Read the model definition and answer for the solid it produces. Units are mm, in the model's axes. A direction names the side the tool comes from. Give positions to 0.01 mm unless a question says otherwise; leave off trailing zeros. Loops run counter-clockwise (first coordinate to the right, second up) from the corner with the lowest first, then second, coordinate; pieces in that order, holes last. Notation, with made-up numbers: (-11.75, 52.5) -> (31.25, 52.5) arc R37 cw to (31.25, 90.5) -> close; hole circle Ø5 at (-34.75, 48). An arc over 180 degrees is marked (long way). Write each question's results on one line, items separated by ' | '. Start each with the question number.
Item 1: Each of these flat-tipped pins is pushed along its axis until it touches: P1, Ø2.5, axis at x = 9.16, y = -37.72, coming from the -Z side; P2, Ø5, axis at x = -6.5, y = -13.5, coming from the -Z side; P3, Ø1.5, axis at y = -6.5, z = 5, coming from the -X side; P4, Ø1.5, axis at y = -25, z = 1.5, coming from the -X side. Where does it stop, or does it pass through?
Item 2: Which of the six approach directions +Z, -Z, +X, -X, +Y, -Y give full straight-line access (tool end or side, diameter ignored) to faces 1 (the flat face through (13.03, 38, 3)), 2 (the cylindrical face through (11.763, -28.375, 2.958))?
Item 3: Section A-A on z = 3.15 is taken. Write down the section's boundary in (x, y), and give its area (3 significant figures).
Item 4: Find the intervals of material crossed by line 1 (Y direction, x = 2.5, z = 3.8); line 2 (Y direction, x = 11, z = 1.1); line 3 (Y direction, x = -7, z = 2.15), in increasing order.
Item 5: Section D-D on x = -4.5 is taken. Write down the section's boundary in (y, z), and give its area (3 significant figures).
Item 6: Section B-B on x = 0 is taken. Write down the section's boundary in (y, z), and give its area (3 significant figures).
Item 7: Section C-C on y = 8.5 is taken. Write down the section's boundary in (x, z).
Autodesk Inventor part; units mm, degrees
ref_plane "YZ Plane" through (0, 0, 0) normal (1, 0, 0) x (0, 1, 0)
ref_plane "XZ Plane" through (0, 0, 0) normal (0, 1, 0) x (-1, 0, 0)
ref_plane "XY Plane" through (0, 0, 0) normal (0, 0, 1) x (1, 0, 0)
sketch "Sketch2" plane through (0, 0, 0) normal (0, 0, 1) x (1, 0, 0)
  line L0 (13.0302, 41.5925) -> (13.0302, -41.5925)
  line L1 (13.0302, -41.5925) -> (-13.0302, -41.5925)
  arc A0 (13.0302, 41.5925) -> (-13.0302, -41.5925) centre (53.0449, -16.618) ccw
  point P0 (0, 0)
  point P1 (13.0302, 0)
  point P2 (0, -41.5925)
  dimension "d6" = 26.0604
  dimension "d32" = 70.6374
  dimension "d33" = 83.185
extrude "Extrusion1" add sketch "Sketch2" along normal blind 6
fillet "Fillet2" radius 7.8 1 edges at (-13.0302, -41.5925, 3)
fillet "Fillet3" radius 4.33 1 edges at (13.0302, -41.5925, 3)
sketch "Sketch6" plane through (0, 0, 6) normal (0, 0, 1) x (1, 0, 0)
  line L0 (13.0302, -37.2625) -> (13.0302, 41.5925)
  arc A0 (8.7002, -41.5925) -> (13.0302, -37.2625) centre (8.7002, -37.2625) ccw
  line L1 (13.0302, -37.2625) -> (13.0302, 41.5925)
  arc A1 (13.0302, 41.5925) -> (-14.9029, -35.9244) centre (53.0449, -16.618) ccw
  arc A2 (-14.9029, -35.9244) -> (-7.3999, -41.5925) centre (-7.3999, -33.7925) ccw
  line L2 (-7.3999, -41.5925) -> (8.7002, -41.5925)
  arc A3 (4.2419, -1.0136) -> (13.0302, -26.6511) centre (10.6426, -13.1445) ccw
  line L3 (13.0302, 0.3621) -> (13.0302, -26.6511)
  arc A4 (13.0302, 23.8159) -> (4.2419, -1.0136) centre (13.0302, 9.8459) ccw
  line L4 (13.0302, 0.3621) -> (13.0302, -4.1241)
  line L5 (13.0302, 0.3621) -> (13.0302, 23.8159)
  point P0 (0, 0)
  dimension "d37" = 2.3876
  dimension "d38" = 13.716
  dimension "d39" = 14.732
  dimension "d41" = 50.8
  dimension "d42" = 13.97
extrude "Extrusion4" cut sketch "Sketch6" against normal through all contours A3 A4 L0
sketch "Sketch7" plane through (0, 0, 6) normal (0, 0, 1) x (1, 0, 0)
  arc A0 (13.0302, 23.8159) -> (4.2419, -1.0136) centre (13.0302, 9.8459) ccw
  line L0 (13.0302, 23.8159) -> (13.0302, 41.5925)
  arc A1 (13.0302, 41.5925) -> (-14.9029, -35.9244) centre (53.0449, -16.618) ccw
  arc A2 (-14.9029, -35.9244) -> (-7.3999, -41.5925) centre (-7.3999, -33.7925) ccw
  line L1 (-7.3999, -41.5925) -> (8.7002, -41.5925)
  arc A3 (8.7002, -41.5925) -> (13.0302, -37.2625) centre (8.7002, -37.2625) ccw
  line L2 (13.0302, -37.2625) -> (13.0302, -26.6511)
  arc A4 (4.2419, -1.0136) -> (13.0302, -26.6511) centre (10.6426, -13.1445) ccw
  line L3 (13.0302, 23.8159) -> (13.0302, 41.5925)
  line L4 (13.0302, 23.8159) -> (17.2669, 23.8159) construction
  arc A5 (13.0302, 36.5159) -> (13.0302, 26.3559) centre (13.0302, 31.4359) ccw
  line L5 (13.0302, 36.5159) -> (13.0302, 26.3559)
  point P0 (0, 0)
  dimension "d46" = 10.16
  dimension "d47" = 2.54
extrude "Extrusion5" cut sketch "Sketch7" against normal through all contours A5 L0
sketch "Sketch8" plane through (0, 0, 6) normal (0, 0, 1) x (1, 0, 0)
  arc A0 (13.0302, 36.5159) -> (13.0302, 26.3559) centre (13.0302, 31.4359) ccw
  line L0 (13.0302, 36.5159) -> (13.0302, 41.5925)
  arc A1 (13.0302, 41.5925) -> (-14.9029, -35.9244) centre (53.0449, -16.618) ccw
  arc A2 (-14.9029, -35.9244) -> (-7.3999, -41.5925) centre (-7.3999, -33.7925) ccw
  line L1 (-7.3999, -41.5925) -> (8.7002, -41.5925)
  arc A3 (8.7002, -41.5925) -> (13.0302, -37.2625) centre (8.7002, -37.2625) ccw
  line L2 (13.0302, -37.2625) -> (13.0302, -26.6511)
  arc A4 (4.2419, -1.0136) -> (13.0302, -26.6511) centre (10.6426, -13.1445) ccw
  arc A5 (13.0302, 23.8159) -> (4.2419, -1.0136) centre (13.0302, 9.8459) ccw
  line L3 (13.0302, 23.8159) -> (13.0302, 26.3559)
  line L4 (13.0302, 39.0559) -> (9.5701, 39.0559)
  arc A6 (13.0302, 41.5925) -> (-14.9029, -35.9244) centre (53.0449, -16.618) ccw
  line L5 (13.0302, 36.5159) -> (13.0302, 41.5925)
  point P0 (0, 0)
  dimension "d50" = 2.54
extrude "Extrusion6" cut sketch "Sketch8" against normal through all contours L4 A1 L0
fillet "Fillet4" radius 5.051 1 edges at (13.0302, -26.6511, 3)
sketch "Sketch9" plane through (0, 0, 6) normal (0, 0, 1) x (1, 0, 0)
  arc A0 (13.0302, -31.7215) -> (8.696, -26.7217) centre (7.9792, -31.7215) ccw
  arc A1 (4.2419, -1.0136) -> (8.696, -26.7217) centre (10.6426, -13.1445) ccw
  arc A2 (13.0302, 23.8159) -> (4.2419, -1.0136) centre (13.0302, 9.8459) ccw
  line L0 (13.0302, 23.8159) -> (13.0302, 26.3559)
  arc A3 (13.0302, 36.5159) -> (13.0302, 26.3559) centre (13.0302, 31.4359) ccw
  arc A4 (9.5701, 39.0559) -> (-14.9029, -35.9244) centre (53.0449, -16.618) ccw
  arc A5 (-14.9029, -35.9244) -> (-7.3999, -41.5925) centre (-7.3999, -33.7925) ccw
  line L1 (-7.3999, -41.5925) -> (8.7002, -41.5925)
  arc A6 (8.7002, -41.5925) -> (13.0302, -37.2625) centre (8.7002, -37.2625) ccw
  line L2 (13.0302, -37.2625) -> (13.0302, -31.7215)
  circle A7 centre (9.1567, -37.719) radius 1.3335
  circle A8 centre (-7.0993, -33.8074) radius 1.8415
  line L3 (13.0302, 36.5159) -> (13.0302, 39.0559)
  line L4 (13.0302, 39.0559) -> (9.5701, 39.0559)
  point P0 (0, 0)
  dimension "d54" = 2.54
  dimension "d55" = 2.54
  dimension "d56" = 2.667
  dimension "d57" = 5.9436
  dimension "d58" = 16.256
  dimension "d59" = 3.683
extrude "Extrusion7" cut sketch "Sketch9" against normal through all contours A7 | A8
properties part number "GripperFingersExtended"
Findings:
1) P1: through | P2: z = 0 | P3: x = -16.97 | P4: x = -17.18
2) face 1: +Z, -Z, +X, +Y, -Y | face 2: +Z, -Z, +X
3) outline: (-14.9, -35.92) arc R7.8 ccw to (-7.4, -41.59) -> (8.7, -41.59) arc R4.33 ccw to (13.03, -37.26) -> (13.03, -31.72) arc R5.05 ccw to (8.7, -26.72) arc R13.72 cw to (4.24, -1.01) arc R13.97 cw to (13.03, 23.82) -> (13.03, 26.36) arc R5.08 cw to (13.03, 36.52) -> (13.03, 39.06) -> (9.57, 39.06) arc R70.64 ccw to start; hole circle Ø3.68 at (-7.1, -33.81); hole circle Ø2.67 at (9.16, -37.72) | area: 1,260 mm2
4) line 1: -41.59 to -24.18, -2.11 to 0.67, 19.03 to 32.73 | line 2: -40.93 to -27.67, 23.67 to 26.78, 36.09 to 39.06 | line 3: -41.59 to -35.65, -31.97 to 20.59
5) outline: (-41.59, 0) -> (24.35, 0) -> (24.35, 6) -> (-41.59, 6) -> close | area: 396 mm2
6) outline: (-41.59, 0) -> (-21.8, 0) -> (-21.8, 6) -> (-41.59, 6) -> close; (-4.49, 0) -> (4.81, 0) -> (4.81, 6) -> (-4.49, 6) -> close; (14.88, 0) -> (30.03, 0) -> (30.03, 6) -> (14.88, 6) -> close | area: 265 mm2
7) outline: (-12.98, 0) -> (-0.87, 0) -> (-0.87, 6) -> (-12.98, 6) -> close
